Part model, mm, in its own coordinate system. Round coordinates to 2 decimals unless told otherwise and drop trailing zeros. Loops run counter-clockwise (first coordinate to the right, second up) from the corner with the lowest first, then second, coordinate; pieces in that order, holes last. Notation, with made-up numbers: (16, 11) -> (71, 11) arc R33 cw to (71, 49) -> close; hole circle Ø3 at (-39, -20.5). An arc over 180 degrees is marked (long way). Use a Markdown table: item, result. Add a question column.
Item 1: Two-plate mould, pull along Z, no slides. Class faces 1 (the face through (5, 5, 300)), 2 (the face through (5, 5, 0)), 3 (the face through (5.1, 5.1, 7.5)): pulls with the +Z half, pulls with the -Z half, needs draft (parallel to the pull), parting line crosses it, or undercut.
Item 2: Probe line 1 (X direction, y = 3.25, z = 10); line 2 (Z direction, x = 5, y = 4); line 3 (Y direction, x = 4.25, z = 144). List the from-to ranges inside material, lowest first. Write a range as [from, to].
Item 3: Cut at A-A, the plane z = 23. List the corners of the cut face in (x, y), plus the area to 3 significant figures.
Item 4: Flat gauge pin, fed straight in: pin 1 (4 mm diameter, centred on x = 9, z = 249.5, fed in from +Y). Where does the tip first touch, or does it go through?
```python
from build123d import *

# Parameters (mm, degrees)
ESQUISSE1_W             = 10
ESQUISSE1_H             = 10
BOSS_EXTRU_1_DEPTH      = 300
ESQUISSE2_R             = 2.5
ENL_V_MAT_EXTRU_1_DEPTH = 301.333148354
ENL_V_MAT_EXTRU_2_DEPTH = 301.333148354
CONG_2_R                = 2
CONG_3_R                = 2
CONG_4_R                = 2


with BuildPart() as part:
    # Esquisse1 → Boss.-Extru.1 (new body)
    with BuildSketch(Plane.XY):
        with Locations((5, 5)):
            Rectangle(ESQUISSE1_W, ESQUISSE1_H)
    extrude(amount=BOSS_EXTRU_1_DEPTH)

    # Esquisse2 → Enlèv. mat.-Extru.1 (cut, through all)
    with BuildSketch(Plane(origin=(0, 10, 0), x_dir=(1, 0, 0), z_dir=(0, 1, 0))):
        with Locations(Location((5, -10, 0), (0, 0, 270))):
            Circle(ESQUISSE2_R)
    extrude(amount=-ENL_V_MAT_EXTRU_1_DEPTH, mode=Mode.SUBTRACT)

    # Esquisse3 → Enlèv. mat.-Extru.2 (cut, through all)
    with BuildSketch(Plane(origin=(0, 0, 0), x_dir=(-1, 0, 0), z_dir=(0, 0, -1))):
        Polygon((0, 10), (0, 8), (-4, 10), align=None)
        Polygon((-10, 10), (-10, 8), (-6, 10), align=None)
    extrude(amount=-ENL_V_MAT_EXTRU_2_DEPTH, mode=Mode.SUBTRACT)

    # Congé2
    cong_2_edges = [part.edges().sort_by_distance(p)[0] for p in [
        (6, 10, 156.145643924),
        (4, 10, 156.145643924),
    ]]
    fillet(cong_2_edges, radius=CONG_2_R)

    # Congé3
    cong_3_edges = [part.edges().sort_by_distance(p)[0] for p in [
        (0, 8, 150),
        (10, 8, 150),
    ]]
    fillet(cong_3_edges, radius=CONG_3_R)

    # Congé4
    cong_4_edges = [part.edges().sort_by_distance(p)[0] for p in [
        (6, 10, 3.854356076),
        (4, 10, 3.854356076),
    ]]
    fillet(cong_4_edges, radius=CONG_4_R)


solid = part.part
```
A:
| question | item | result |
|---|---|---|
| 1 | face 1 | pulls with the +Z half |
| 1 | face 2 | pulls with the -Z half |
| 1 | face 3 | undercut |
| 2 | line 1 | x = [0, 2.5], [7.5, 10] |
| 2 | line 2 | z = [0, 7.5], [12.5, 300] |
| 2 | line 3 | y = [0, 9.99] |
| 3 | outline | (0, 0) -> (10, 0) -> (10, 6.76) arc R2 ccw to (8.89, 8.55) -> (6.42, 9.79) arc R2 ccw to (5.53, 10) -> (4.47, 10) arc R2 ccw to (3.58, 9.79) -> (1.11, 8.55) arc R2 ccw to (0, 6.76) -> close |
| 3 | area | 91.5 mm^2 |
| 4 | pin 1 | stops at y = 9.5 |
